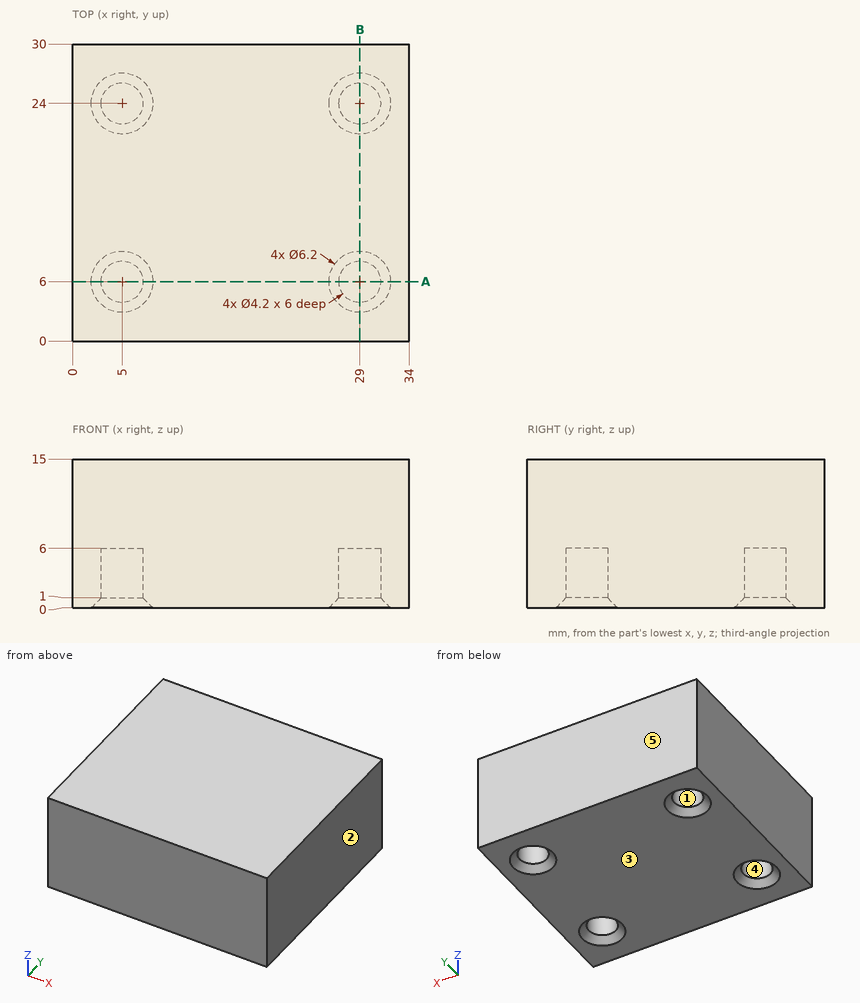
Part print with two shaded views. Sizes in mm from the minimum x, y, z corner. A direction names the side the tool comes from. Coordinates: 2 decimals unless noted, no trailing zeros. Write each loop counter-clockwise with the first axis right and the second up, starting at its lowest first coordinate (ties: lowest second). Pieces come first, ordered by that corner, then holes. Notation, with made-up numbers: M 69.5,19 L 124.5,19 A17 ccw 124.5,40 Z; hole C 79,-7 d10. An arc over 180 degrees is marked long. Return JSON: item names as keys, results as strings.
Item 1: Slice it at A-A, the plane y = 6. Write the cut outline in (x, z).
Findings below:
{"outline": "M 0,0 L 1.9,0 L 2.9,1 L 2.9,6 L 7.1,6 L 7.1,1 L 8.1,0 L 25.9,0 L 26.9,1 L 26.9,6 L 31.1,6 L 31.1,1 L 32.1,0 L 34,0 L 34,15 L 0,15 Z"}
Item 2: Drop flat-ended pins along their axis: pin 1 Ø3.5 at (x, y) = (4.5, 6) entering from -Z; pin 2 Ø2 at (x, y) = (29, 6) entering from -Z; pin 3 Ø5 at (x, y) = (29, 6) entering from -Z. Give the stop position or say it passes through.
Findings below:
{"pin 1": "stops at z = 0.85", "pin 2": "stops at z = 6", "pin 3": "stops at z = 0.6"}
Item 3: Which spindle directions (+Z, -Z, +X, -X, +Y, -Y) get a long thin tool onto all of the face, cutting with end or side? Do the marked faces 1 and 2. Say none if no direction does.
Findings below:
{"face 1": "-Z", "face 2": "+Z, -Z, +X, +Y, -Y"}
Item 4: Probe line 1 (Y direction, x = 29, z = 3.1); line 2 (Z direction, x = 31, y = 8.25); line 3 (Z direction, x = 5, y = 3.25). List the from-to ranges inside material, lowest first. Write a range as from..to.
Findings below:
{"line 1": "y = 0..3.9, 8.1..21.9, 26.1..30", "line 2": "z = 0.09..15", "line 3": "z = 0.35..15"}
Item 5: Slice it at B-B, the plane x = 29. Write the cut outline in (y, z).
Findings below:
{"outline": "M 0,0 L 2.9,0 L 3.9,1 L 3.9,6 L 8.1,6 L 8.1,1 L 9.1,0 L 20.9,0 L 21.9,1 L 21.9,6 L 26.1,6 L 26.1,1 L 27.1,0 L 30,0 L 30,15 L 0,15 Z"}
Item 6: Two-plate mould, pull along Y, no slides. Class the marked faces 3, 4 and 5: +Y half, -Y half, draft (parallel to the pull), parting line (faces both ways), or undercut.
Findings below:
{"face 3": "draft", "face 4": "undercut", "face 5": "+Y half"}
